The listing builds one solid part. Answer for the finished solid, in the listing's coordinates (mm). A direction names the side the tool comes from. Coordinates: 2 decimals unless noted, no trailing zeros. Order: outer loops, then holes, each group sorted by start corner. A loop starts at its lowest first (then second) coordinate and runs counter-clockwise, first axis right, second up. Notation, with made-up numbers: (37, 3.5) - (85, 3.5) arc R24 cw to (85, 39.5) - close; hole circle Ø9 at (20.5, 74). An arc over 180 degrees is marked (long way). Use a Markdown table: item, result. Add a question column.
Item 1: The part is cut by section B-B, the plane y = 16.5. Give the vertices of the cut face in (x, z), then the cut area to 4 significant figures.
Item 2: The part is cut by section A-A, the plane z = 86.5. Give the vertices of the cut face in (x, y), then the cut area to 3 significant figures.
Item 3: For faces 1 (the flat face through (1, 79.284, 77)), 2 (the flat face through (1, 63, 24.699)), determine the directions among +Z, -Z, +X, -X, +Y, -Y from which every point of the face is accessible in a straight line to the end or side of a thin tool.
Item 4: The part is cut by section C-C, the plane z = 34. Give the vertices of the cut face in (x, y).
Item 5: The mould has two halves that part along Y. Classify faces 3 (the flat face through (1, 9.974, 78)), 4 (the flat face through (1, 4.284, 79)), 5 (the flat face through (0, 41, 79)), 6 (the flat face through (1, 20, 131.919)): released by +Y, released by -Y, zero draft, split by the parting line, or undercut.
Item 6: Find the intervals of material crossed by line 1 along Y through (x, z) = (0.45, 28); line 2 along Z through (x, y) = (0.4, 71.5); line 3 along Y through (x, z) = (0.7, 89), in increasing order.
Item 7: The part is cut by section D-D, the plane x = 1.05. Give the vertices of the cut face in (y, z).
from build123d import *

# Parameters (mm, degrees)
F0_W     = 13.9900064
F0_H     = 3.81
F0_W_2   = 21
F0_H_2   = 21
F1_DEPTH = 2.5


# Not quite as in the source:
# - a feature names something its author has since deleted; it is built from what else it names


with BuildPart() as f1:
    # F0 (on Right) → F1 (new body)
    with BuildSketch(Plane.YZ):
        Polygon((4.2842663067, 140.8092032793), (4.2842663067, 15.8092032793), (79.2842663067, 15.8092032793), (79.2842663067, 140.8092032793), (75.4742663067, 140.8092032793), (75.4742663067, 136.9992032793), (75.4742663067, 19.6192032793), (8.0942663067, 19.6192032793), (8.0942663067, 136.9992032793), (55.7998448917, 136.9992032793), (61.4842599067, 136.9992032793), (61.4842599067, 140.8092032793), (55.7998448917, 140.8092032793), (11.2942599067, 140.8092032793), align=None)
        with Locations((68.4792631067, 138.9042032793)):
            Rectangle(F0_W, F0_H)
        Polygon((75.4742663067, 19.6192032793), (75.4742663067, 136.9992032793), (61.4842599067, 136.9992032793), (55.7998448917, 136.9992032793), (8.0942663067, 136.9992032793), (8.0942663067, 19.6192032793), align=None)
        Polygon((9.9742727067, 45.6992032793), (9.9742727067, 131.9192032793), (30.9742727067, 131.9192032793), (30.9742727067, 110.9192032793), (30.9742727067, 45.6992032793), (30.9742727067, 24.6992032793), (9.9742727067, 24.6992032793), align=None, mode=Mode.SUBTRACT)
        with Locations((63.0942599067, 35.1992032793)):
            Rectangle(F0_W_2, F0_H_2, mode=Mode.SUBTRACT)
    extrude(amount=F1_DEPTH)


solid = f1.part
Solution:
| question | item | result |
|---|---|---|
| 1 | outline | (0, 15.81) - (2.5, 15.81) - (2.5, 24.7) - (0, 24.7) - close; (0, 131.92) - (2.5, 131.92) - (2.5, 140.81) - (0, 140.81) - close |
| 1 | area | 44.45 mm2 |
| 2 | outline | (0, 4.28) - (2.5, 4.28) - (2.5, 9.97) - (0, 9.97) - close; (0, 30.97) - (2.5, 30.97) - (2.5, 79.28) - (0, 79.28) - close |
| 2 | area | 135 mm2 |
| 3 | face 1 | +Z, -Z, +X, -X, +Y |
| 3 | face 2 | +X, -X |
| 4 | outline | (0, 4.28) - (2.5, 4.28) - (2.5, 9.97) - (0, 9.97) - close; (0, 30.97) - (2.5, 30.97) - (2.5, 52.59) - (0, 52.59) - close; (0, 73.59) - (2.5, 73.59) - (2.5, 79.28) - (0, 79.28) - close |
| 5 | face 3 | undercut |
| 5 | face 4 | released by -Y |
| 5 | face 5 | zero draft |
| 5 | face 6 | undercut |
| 6 | line 1 | y = 4.28 to 9.97, 30.97 to 52.59, 73.59 to 79.28 |
| 6 | line 2 | z = 15.81 to 24.7, 45.7 to 140.81 |
| 6 | line 3 | y = 4.28 to 9.97, 30.97 to 79.28 |
| 7 | outline | (4.28, 15.81) - (79.28, 15.81) - (79.28, 140.81) - (4.28, 140.81) - close; hole (9.97, 24.7) - (30.97, 24.7) - (30.97, 131.92) - (9.97, 131.92) - close; hole (52.59, 24.7) - (73.59, 24.7) - (73.59, 45.7) - (52.59, 45.7) - close |
